from build123d import *

# Parameters (mm, degrees)
SKETCH1_W            = 50
SKETCH1_H            = 30
BASE_FLANGE1_DEPTH   = 1.51892
EDGE_FLANGE1_DEPTH   = 50
M8_CLEARANCE_HOLE1_D = 9
CUT_EXTRUDE1_DEPTH   = 55.277389816


# Sheet-metal steps are written as plain solids
with BuildPart() as part:
    # Sketch1 → Base-Flange1 (new body)
    with BuildSketch(Plane(origin=(0, 0, 0), x_dir=(1, 0, 0), z_dir=(0, 1, 0))):
        with Locations((0, 15)):
            Rectangle(SKETCH1_W, SKETCH1_H)
    extrude(amount=BASE_FLANGE1_DEPTH)

    # Edge-Flange1 section (across the edge) → Edge-Flange1 (add)
    with BuildSketch(Plane(origin=(-25, 1.51892, 1.5875), x_dir=(0, 0, -1), z_dir=(1, 0, 0))):
        with BuildLine():
            Line((-1.51892, 1.5875), (-1.51892, 33.48108))
            Line((-1.51892, 33.48108), (0, 33.48108))
            Line((0, 33.48108), (0, 1.5875))
            ThreePointArc((0, 1.5875), (0.464967985, 0.464967985), (1.5875, 0))
            Line((1.5875, 0), (1.5875, -1.51892))
            ThreePointArc((1.5875, -1.51892), (-0.609070647, -0.609070647), (-1.51892, 1.5875))
        make_face()
    extrude(amount=EDGE_FLANGE1_DEPTH)

    # M8 Clearance Hole1 (through all)
    with Locations(Plane(origin=(0, 1.51892, 0), x_dir=(1, 0, 0), z_dir=(0, 1, 0))):
        with Locations((-13, 21.89358)):
            Hole(M8_CLEARANCE_HOLE1_D / 2)

    # Sketch11 → Cut-Extrude1 (cut, through all)
    with BuildSketch(Plane.XY.offset(3.10642)):
        with BuildLine():
            Line((-0.536205236, 33.346354167), (-0.536205236, 31.25))
            add(Edge.make_bspline(
                [(-0.536205236, 31.25), (-0.732304351, 31.187728797), (-1.102067969, 31.070310494), (-1.604733174, 30.833115296), (-2.017508244, 30.547560299), (-2.348134384, 30.212441135), (-2.583648684, 29.809655364), (-2.755765248, 29.34801065), (-2.848017529, 28.810847769), (-2.862096707, 28.430876813), (-2.869538569, 28.230034722)],
                knots=[0, 0, 0, 0, 1.177836724, 2.220923683, 3.170508287, 4.04032801, 4.893978525, 5.822851288, 6.849219673, 8, 8, 8, 8], degree=3))
            Line((-2.869538569, 28.230034722), (-2.869538569, 9.490451389))
            add(Edge.make_bspline(
                [(-2.869538569, 9.490451389), (-2.867825411, 9.340569917), (-2.864676289, 9.065058229), (-2.856032947, 8.687922323), (-2.830901599, 8.38587715), (-2.796864936, 8.086599995), (-2.694246063, 7.767569857), (-2.532312838, 7.572117956), (-2.450267736, 7.473090278)],
                knots=[0, 0, 0, 0, 1.276365713, 2.34621177, 3.211297358, 3.855222149, 4.913326661, 6, 6, 6, 6], degree=3))
            add(Edge.make_bspline(
                [(-2.450267736, 7.473090278), (-2.372143104, 7.400138444), (-2.201489167, 7.240783867), (-1.849576421, 7.073415225), (-1.421039194, 6.915571991), (-1.09843104, 6.839489909), (-0.925094125, 6.798611111)],
                knots=[0, 0, 0, 0, 0.755126351, 1.649483421, 2.737070691, 4, 4, 4, 4], degree=3))
            Line((-0.925094125, 6.798611111), (-0.925094125, 4.659722222))
            add(Edge.make_bspline(
                [(-0.925094125, 4.659722222), (-1.254477967, 4.70572391), (-1.909616136, 4.797220389), (-2.867595341, 5.052416526), (-3.795873677, 5.392904571), (-4.688251224, 5.825940849), (-5.545074878, 6.341217745), (-6.343237475, 6.957264962), (-7.115245839, 7.634651596), (-7.571961107, 8.152383248), (-7.803566347, 8.414930556)],
                knots=[0, 0, 0, 0, 0.993273036, 1.975601091, 2.956248835, 3.944528193, 4.936047062, 5.938575079, 6.95462918, 8, 8, 8, 8], degree=3))
            add(Edge.make_bspline(
                [(-7.803566347, 8.414930556), (-8.055058907, 8.733178871), (-8.569676873, 9.384396149), (-9.198622321, 10.4993388), (-9.754805445, 11.72710012), (-10.215414522, 13.070861325), (-10.585289747, 14.50493195), (-10.841878152, 16.009183271), (-11.005265617, 17.572495268), (-11.025763903, 18.635000654), (-11.036205236, 19.176215278)],
                knots=[0, 0, 0, 0, 0.848908429, 1.737083309, 2.673598995, 3.670958022, 4.709700774, 5.773871062, 6.866063596, 8, 8, 8, 8], degree=3))
            add(Edge.make_bspline(
                [(-11.036205236, 19.176215278), (-11.026382584, 19.748044697), (-11.00719909, 20.864819137), (-10.803957186, 22.492136825), (-10.496270468, 24.032412225), (-10.041921928, 25.477668954), (-9.472269882, 26.8365081), (-8.767858972, 28.100340729), (-7.942830537, 29.28019574), (-7.291562466, 29.981060383), (-6.96502468, 30.332465278)],
                knots=[0, 0, 0, 0, 1.125083173, 2.197270879, 3.223201206, 4.213147336, 5.174373174, 6.118528402, 7.056653326, 8, 8, 8, 8], degree=3))
            add(Edge.make_bspline(
                [(-6.96502468, 30.332465278), (-6.725570757, 30.561318773), (-6.251387297, 31.014510524), (-5.487846636, 31.614362799), (-4.688422822, 32.12911505), (-3.86871675, 32.565937556), (-3.032292491, 32.912249239), (-2.196660266, 33.165240479), (-1.364102414, 33.317178289), (-0.810236123, 33.33669706), (-0.536205236, 33.346354167)],
                knots=[0, 0, 0, 0, 1.091574889, 2.161613191, 3.195169959, 4.222755612, 5.219792993, 6.174728054, 7.096928445, 8, 8, 8, 8], degree=3))
        make_face()
        with BuildLine():
            Line((1.01935032, 31.25), (1.01935032, 33.346354167))
            add(Edge.make_bspline(
                [(1.01935032, 33.346354167), (1.35638191, 33.334410674), (2.037279483, 33.310281496), (3.058991771, 33.118596613), (4.086623836, 32.809565238), (4.751119346, 32.513303808), (5.090530875, 32.361979167)],
                knots=[0, 0, 0, 0, 0.957329974, 1.934072875, 2.94476415, 4, 4, 4, 4], degree=3))
            add(Edge.make_bspline(
                [(5.090530875, 32.361979167), (5.37000628, 32.21892083), (5.91492361, 31.939987638), (6.646983826, 31.416730734), (7.286526768, 30.837752524), (7.82321414, 30.197129791), (8.256096639, 29.513712062), (8.573154519, 28.794283899), (8.762120848, 28.043236683), (8.785435523, 27.532288153), (8.797128098, 27.276041667)],
                knots=[0, 0, 0, 0, 1.133386976, 2.209862454, 3.240979251, 4.243853893, 5.220771738, 6.155072333, 7.074747837, 8, 8, 8, 8], degree=3))
            add(Edge.make_bspline(
                [(8.797128098, 27.276041667), (8.785638647, 27.003188082), (8.763244087, 26.471357992), (8.548147846, 25.708802292), (8.197928052, 25.014727339), (7.708022484, 24.411080511), (7.125276809, 23.904679385), (6.45424304, 23.538240792), (5.711854464, 23.317351012), (5.193341007, 23.291224684), (4.926468375, 23.277777778)],
                knots=[0, 0, 0, 0, 1.052335015, 2.051149251, 3.034759759, 4.037094461, 5.036307284, 5.99952726, 6.970380773, 8, 8, 8, 8], degree=3))
            add(Edge.make_bspline(
                [(4.926468375, 23.277777778), (4.690324716, 23.288887346), (4.228795332, 23.310600367), (3.563454835, 23.498531551), (2.960039675, 23.816514126), (2.421279895, 24.239764216), (1.97438813, 24.750484649), (1.643916355, 25.323376327), (1.446805269, 25.950992233), (1.421287465, 26.385472211), (1.408239209, 26.607638889)],
                knots=[0, 0, 0, 0, 1.052177608, 2.056421433, 3.054792914, 4.078048738, 5.096504648, 6.06384139, 7.009966053, 8, 8, 8, 8], degree=3))
            add(Edge.make_bspline(
                [(1.408239209, 26.607638889), (1.417230139, 26.788519635), (1.435506133, 27.156198562), (1.561436361, 27.705294624), (1.770484915, 28.252331108), (1.964711734, 28.598881271), (2.064489209, 28.776909722)],
                knots=[0, 0, 0, 0, 0.946230724, 1.923416974, 2.933225545, 4, 4, 4, 4], degree=3))
            add(Edge.make_bspline(
                [(2.064489209, 28.776909722), (2.152068669, 28.919314407), (2.30090363, 29.161320873), (2.46871514, 29.496928508), (2.563747337, 29.786024985), (2.571152453, 29.971229688), (2.574905875, 30.065104167)],
                knots=[0, 0, 0, 0, 1.426676034, 2.424532782, 3.201444875, 4, 4, 4, 4], degree=3))
            add(Edge.make_bspline(
                [(2.574905875, 30.065104167), (2.57089384, 30.142783896), (2.563194833, 30.291849587), (2.484310793, 30.502479258), (2.358514484, 30.688139304), (2.186764713, 30.855164059), (1.959059048, 30.986654466), (1.690482224, 31.102662213), (1.371607963, 31.192747437), (1.141356267, 31.230170329), (1.01935032, 31.25)],
                knots=[0, 0, 0, 0, 0.864688311, 1.659317839, 2.475251474, 3.355494564, 4.310252246, 5.394837407, 6.619574429, 8, 8, 8, 8], degree=3))
        make_face()
        with BuildLine():
            Line((-0.925094125, 17.748263889), (-0.925094125, 20.105902778))
            add(Edge.make_bspline(
                [(-0.925094125, 20.105902778), (-0.562172057, 20.292252137), (0.141848053, 20.653744887), (1.229104149, 21.047376471), (2.303547114, 21.282260708), (3.015380537, 21.316516402), (3.364836431, 21.333333333)],
                knots=[0, 0, 0, 0, 1.085282539, 2.105302489, 3.069848097, 4, 4, 4, 4], degree=3))
            add(Edge.make_bspline(
                [(3.364836431, 21.333333333), (3.575767493, 21.32728003), (3.999566405, 21.315117842), (4.635355291, 21.222102337), (5.267804942, 21.05982284), (5.896889917, 20.850033552), (6.507494748, 20.584589713), (7.083966485, 20.267929702), (7.626171736, 19.909707688), (7.95313475, 19.631336083), (8.116572542, 19.4921875)],
                knots=[0, 0, 0, 0, 0.972589152, 1.954108701, 2.955474046, 3.980479148, 5.009562198, 6.021200449, 7.010864794, 8, 8, 8, 8], degree=3))
            add(Edge.make_bspline(
                [(8.116572542, 19.4921875), (8.286591287, 19.323607302), (8.627940088, 18.985146688), (9.071361238, 18.408935486), (9.454453028, 17.780658412), (9.776451155, 17.106691604), (10.028216962, 16.397029145), (10.222125832, 15.662485068), (10.331364306, 14.901746379), (10.345542817, 14.386322918), (10.352683653, 14.126736111)],
                knots=[0, 0, 0, 0, 0.960654025, 1.928717332, 2.91079185, 3.911286876, 4.922404946, 5.930508659, 6.95772566, 8, 8, 8, 8], degree=3))
            add(Edge.make_bspline(
                [(10.352683653, 14.126736111), (10.342759002, 13.779655432), (10.322905808, 13.085357977), (10.142569288, 12.051162813), (9.862554364, 11.02542886), (9.476763198, 10.022432767), (9.004721612, 9.072584195), (8.453195982, 8.205333864), (7.831858662, 7.432367139), (7.350754184, 6.995429904), (7.113968375, 6.780381944)],
                knots=[0, 0, 0, 0, 1.007304958, 2.015004901, 3.039646456, 4.091698815, 5.130844098, 6.114845671, 7.072181175, 8, 8, 8, 8], degree=3))
            add(Edge.make_bspline(
                [(7.113968375, 6.780381944), (6.90801948, 6.620680668), (6.492761858, 6.298672764), (5.810841905, 5.877851847), (5.075224903, 5.510264937), (4.300519423, 5.189578578), (3.502536323, 4.938418331), (2.707743298, 4.746095899), (1.917876024, 4.633000789), (1.394402127, 4.618367855), (1.134801709, 4.611111111)],
                knots=[0, 0, 0, 0, 0.965288144, 1.946323901, 2.963451572, 4.010279453, 5.050032815, 6.060491454, 7.038161726, 8, 8, 8, 8], degree=3))
            Line((1.134801709, 4.611111111), (0.630461431, 4.659722222))
            Line((0.630461431, 4.659722222), (0.630461431, 6.798611111))
            add(Edge.make_bspline(
                [(0.630461431, 6.798611111), (0.761629372, 6.832809064), (1.009712074, 6.897488897), (1.339469946, 7.055085592), (1.619820156, 7.225387633), (1.836416232, 7.442876654), (2.00089705, 7.701001552), (2.10558164, 8.011490131), (2.173038554, 8.367464004), (2.181530549, 8.621171288), (2.186016987, 8.755208333)],
                knots=[0, 0, 0, 0, 1.174511043, 2.221395497, 3.163228448, 4.009149245, 4.86326273, 5.798169132, 6.836742493, 8, 8, 8, 8], degree=3))
            Line((2.186016987, 8.755208333), (2.186016987, 16.387152778))
            add(Edge.make_bspline(
                [(2.186016987, 16.387152778), (2.181817499, 16.525217563), (2.17384572, 16.787302382), (2.101574404, 17.159744372), (1.974463868, 17.485857622), (1.796962527, 17.761186859), (1.584899926, 17.984342452), (1.334196604, 18.144788488), (1.046391899, 18.224495567), (0.847588512, 18.222991473), (0.74591282, 18.222222222)],
                knots=[0, 0, 0, 0, 1.252532866, 2.377650834, 3.425917608, 4.410309965, 5.333554112, 6.20090564, 7.079874001, 8, 8, 8, 8], degree=3))
            add(Edge.make_bspline(
                [(0.74591282, 18.222222222), (0.630014522, 18.213015719), (0.379223237, 18.193093849), (-0.016789147, 18.093798205), (-0.460026427, 17.948951586), (-0.764057901, 17.817754823), (-0.925094125, 17.748263889)],
                knots=[0, 0, 0, 0, 0.797685093, 1.726103611, 2.795586252, 4, 4, 4, 4], degree=3))
        make_face()
    extrude(amount=-CUT_EXTRUDE1_DEPTH, mode=Mode.SUBTRACT)


solid = part.part
For this review, take the finished solid that the model builds, in its own axes (mm). A direction names the side the tool comes from. Give positions to 0.01 mm unless a question says otherwise; leave off trailing zeros. Order: outer loops, then holes, each group sorted by start corner. A loop starts at its lowest first (then second) coordinate and runs counter-clockwise, first axis right, second up. Notation, with made-up numbers: M -11.75,46.5 L -4.75,46.5 A29 ccw -4.75,67.5 Z; hole C 27.25,73.25 d3. An arc over 180 degrees is marked long. Answer in a Markdown table with one row per item. Add a question column.
(1) Consider section C-C on x = -18.5. State the section outline as (y, z) points (1 decimal), and give its area (3 significant figures).
(2) Mouldability with a two-part tool opening along X and no side actions: class faces 4 (the face through (-0.536, 32, 2)), 5 (the face through (0, 22, 3.106)), 6 (the face through (25, 10, 2)), 7 (the face through (-25, 10, 2)) as +X half, -X half, draft (parallel to the pull), parting line (faces both ways), or undercut.
(3) Consider section D-D on z = -8.5. State the section outline as (x, y) points, and give its area (3 significant figures).
(4) Consider section B-B on z = -20. State the section outline as (x, y) points.
(5) Wall thickness on probe 1 along Y at (x, z) = (19.5, -9.5); probe 2 along Z at (x, y) = (12.5, 23); probe 3 along Z at (x, y) = (-13, 1.1): over which ranges is each line inside the solid? List them lowest first. Write a range as [from, to].
(6) Consider section A-A on x = -13. State the section outline as (y, z) points (1 decimal).
(7) For pin 1 (6 mm diameter, centred on x = -17, y = 29.5, fed in from -Z); pin 2 (15 mm diameter, centred on x = 4, z = -11, fed in from +Y); pin 3 (2 mm diameter, centred on x = -5, y = 31, fed in from +Z), all flat-tipped, find the tip position at first contact; note any pin that passes through.
(8) For faces 1 (the face through (-17.29, 0.75, -23.25)), 2 (the face through (2.186, 13, 2)), 3 (the face through (0, 23, 1.588)), list the 3-axis set-ups (+Z, -Z, +X, -X, +Y, -Y) from which the entire face can be reached by the end or side of a thin tool; tool diameter is ignored.
Evaluation:
| question | item | result |
|---|---|---|
| 1 | outline | M 0,-30 L 1.5,-30 L 1.5,0 A1.6 cw 3.1,1.6 L 35,1.6 L 35,3.1 L 3.1,3.1 A3.1 ccw 0,0 Z |
| 1 | area | 99.6 mm^2 |
| 2 | face 4 | undercut |
| 2 | face 5 | draft |
| 2 | face 6 | +X half |
| 2 | face 7 | -X half |
| 3 | outline | M -25,0 L 25,0 L 25,1.52 L -25,1.52 Z |
| 3 | area | 75.9 mm^2 |
| 4 | outline | M -25,0 L -17.08,0 L -17.08,1.52 L -25,1.52 Z; M -8.92,0 L 25,0 L 25,1.52 L -8.92,1.52 Z |
| 5 | probe 1 | y = [0, 1.52] |
| 5 | probe 2 | z = [1.59, 3.11] |
| 5 | probe 3 | z = [-30, -26.39], [-17.39, 2.37] |
| 6 | outline | M 0,-30 L 1.5,-30 L 1.5,-26.4 L 0,-26.4 Z; M 0,-17.4 L 1.5,-17.4 L 1.5,0 A1.6 cw 3.1,1.6 L 35,1.6 L 35,3.1 L 3.1,3.1 A3.1 ccw 0,0 Z |
| 7 | pin 1 | stops at z = 1.59 |
| 7 | pin 2 | stops at y = 1.52 |
| 7 | pin 3 | stops at z = 3.11 |
| 8 | face 1 | +Y, -Y |
| 8 | face 2 | +Z, -Z |
| 8 | face 3 | -Z, +X, -X, +Y |
